For this review, take the finished solid that the model builds, in its own axes (mm). Round coordinates to 2 decimals unless told otherwise and drop trailing zeros. Loops run counter-clockwise (first coordinate to the right, second up) from the corner with the lowest first, then second, coordinate; pieces in that order, holes last.
1. Clearance check with a flat-ended pin moving along its axis: pin 1 Ø4 at (x, y) = (174.625, -53.975) entering from +Z. State where the tip first meets the part, or that it passes through.
2. Draft analysis for pull direction X (two halves, no side actions). For faces 1 (the cylindrical face through (176.971, -13.673, 1.288)), 2 (the flat face through (91, -74, 0)), state which applies: released by +X, released by -X, zero draft, split by the parting line, or undercut.
3. Consider section A-A on y = -95.25. State the section outline as (x, z) points (3 decimals).
4. To check wall thickness, follow line 1 along X through (y, z) = (-53.5, 2.15); line 2 along Y through (x, z) = (11.5, 0.55) (3 decimals); line 3 along Y through (x, z) = (11, 0.95) (3 decimals). State the ranges of each line that lie inside material, in increasing order.
from build123d import *

# Parameters (mm, degrees)
SKETCH1_W                 = 184.15
SKETCH1_H                 = 149.225
BOSS_EXTRUDE1_DEPTH       = 2.54
SKETCH2_R                 = 2.54
CUT_EXTRUDE1_DEPTH        = 2.54
LPATTERN1_COUNT           = 2
LPATTERN1_PITCH           = 50.8
LPATTERN2_COUNT           = 2
LPATTERN2_PITCH           = 41.275
LPATTERN2_COPY_1_SKETCH_R = 2.54
LPATTERN2_COPY_1_DEPTH    = 2.54
SKETCH3_R                 = 2.54
CUT_EXTRUDE2_DEPTH        = 2.54
LPATTERN3_COUNT           = 2
LPATTERN3_PITCH           = 50.8
LPATTERN4_COUNT           = 2
LPATTERN4_PITCH           = 41.275
LPATTERN4_COPY_1_SKETCH_R = 2.54
LPATTERN4_COPY_1_DEPTH    = 2.54
SKETCH5_R                 = 2.54
CUT_EXTRUDE4_DEPTH        = 2.54
LPATTERN7_COUNT           = 2
LPATTERN7_PITCH           = 41.275
LPATTERN8_COUNT           = 2
LPATTERN8_PITCH           = 50.8
LPATTERN8_COPY_1_SKETCH_R = 2.54
LPATTERN8_COPY_1_DEPTH    = 2.54
LPATTERN9_COUNT           = 2
LPATTERN9_PITCH           = 82.55
LPATTERN9_COPY_1_SKETCH_R = 2.54
LPATTERN9_COPY_1_DEPTH    = 2.54
LPATTERN9_COPY_2_SKETCH_R = 2.54
LPATTERN9_COPY_2_DEPTH    = 2.54
LPATTERN9_COPY_3_SKETCH_R = 2.54
LPATTERN9_COPY_3_DEPTH    = 2.54


with BuildPart() as part:
    # Sketch1 → Boss-Extrude1 (new body)
    with BuildSketch(Plane.XY):
        with Locations((92.075, -74.6125)):
            Rectangle(SKETCH1_W, SKETCH1_H)
    extrude(amount=BOSS_EXTRUDE1_DEPTH)

    # Sketch2 → Cut-Extrude1 (cut)
    with BuildSketch(Plane.XY.offset(2.54)):
        with Locations((9.525, -12.7)):
            Circle(SKETCH2_R)
    cut_extrude1 = extrude(amount=-CUT_EXTRUDE1_DEPTH, mode=Mode.SUBTRACT)

    # LPattern1: Cut-Extrude1 ×2
    with Locations(*[(i * LPATTERN1_PITCH, 0, 0) for i in range(1, LPATTERN1_COUNT)]):
        add(cut_extrude1, mode=Mode.SUBTRACT)

    # LPattern2: Cut-Extrude1 ×2
    with Locations(*[(0, -i * LPATTERN2_PITCH, 0) for i in range(1, LPATTERN2_COUNT)]):
        add(cut_extrude1, mode=Mode.SUBTRACT)

    # LPattern2 copy 1 sketch → LPattern2 copy 1 (cut)
    with BuildSketch(Plane(origin=(50.8, -41.275, 2.54), x_dir=(1, 0, 0), z_dir=(0, 0, 1))):
        with Locations((9.525, -12.7)):
            Circle(LPATTERN2_COPY_1_SKETCH_R)
    extrude(amount=-LPATTERN2_COPY_1_DEPTH, mode=Mode.SUBTRACT)

    # Sketch3 → Cut-Extrude2 (cut)
    with BuildSketch(Plane.XY.offset(2.54)):
        with Locations((123.825, -12.7)):
            Circle(SKETCH3_R)
    cut_extrude2 = extrude(amount=-CUT_EXTRUDE2_DEPTH, mode=Mode.SUBTRACT)

    # LPattern3: Cut-Extrude2 ×2
    with Locations(*[(i * LPATTERN3_PITCH, 0, 0) for i in range(1, LPATTERN3_COUNT)]):
        add(cut_extrude2, mode=Mode.SUBTRACT)

    # LPattern4: Cut-Extrude2 ×2
    with Locations(*[(0, -i * LPATTERN4_PITCH, 0) for i in range(1, LPATTERN4_COUNT)]):
        add(cut_extrude2, mode=Mode.SUBTRACT)

    # LPattern4 copy 1 sketch → LPattern4 copy 1 (cut)
    with BuildSketch(Plane(origin=(50.8, -41.275, 2.54), x_dir=(1, 0, 0), z_dir=(0, 0, 1))):
        with Locations((123.825, -12.7)):
            Circle(LPATTERN4_COPY_1_SKETCH_R)
    extrude(amount=-LPATTERN4_COPY_1_DEPTH, mode=Mode.SUBTRACT)

    # Sketch5 → Cut-Extrude4 (cut)
    with BuildSketch(Plane.XY.offset(2.54)):
        with Locations((9.525, -136.525)):
            Circle(SKETCH5_R)
    cut_extrude4 = extrude(amount=-CUT_EXTRUDE4_DEPTH, mode=Mode.SUBTRACT)

    # LPattern7: Cut-Extrude4 ×2
    with Locations(*[(0, i * LPATTERN7_PITCH, 0) for i in range(1, LPATTERN7_COUNT)]):
        add(cut_extrude4, mode=Mode.SUBTRACT)

    # LPattern8: Cut-Extrude4 ×2
    with Locations(*[(i * LPATTERN8_PITCH, 0, 0) for i in range(1, LPATTERN8_COUNT)]):
        add(cut_extrude4, mode=Mode.SUBTRACT)

    # LPattern8 copy 1 sketch → LPattern8 copy 1 (cut)
    with BuildSketch(Plane(origin=(50.8, 41.275, 2.54), x_dir=(1, 0, 0), z_dir=(0, 0, 1))):
        with Locations((9.525, -136.525)):
            Circle(LPATTERN8_COPY_1_SKETCH_R)
    extrude(amount=-LPATTERN8_COPY_1_DEPTH, mode=Mode.SUBTRACT)

    # LPattern9: Cut-Extrude2 ×2
    with Locations(*[(0, -i * LPATTERN9_PITCH, 0) for i in range(1, LPATTERN9_COUNT)]):
        add(cut_extrude2, mode=Mode.SUBTRACT)

    # LPattern9 copy 1 sketch → LPattern9 copy 1 (cut)
    with BuildSketch(Plane(origin=(50.8, -82.55, 2.54), x_dir=(1, 0, 0), z_dir=(0, 0, 1))):
        with Locations((123.825, -12.7)):
            Circle(LPATTERN9_COPY_1_SKETCH_R)
    extrude(amount=-LPATTERN9_COPY_1_DEPTH, mode=Mode.SUBTRACT)

    # LPattern9 copy 2 sketch → LPattern9 copy 2 (cut)
    with BuildSketch(Plane(origin=(0, -123.825, 2.54), x_dir=(1, 0, 0), z_dir=(0, 0, 1))):
        with Locations((123.825, -12.7)):
            Circle(LPATTERN9_COPY_2_SKETCH_R)
    extrude(amount=-LPATTERN9_COPY_2_DEPTH, mode=Mode.SUBTRACT)

    # LPattern9 copy 3 sketch → LPattern9 copy 3 (cut)
    with BuildSketch(Plane(origin=(50.8, -123.825, 2.54), x_dir=(1, 0, 0), z_dir=(0, 0, 1))):
        with Locations((123.825, -12.7)):
            Circle(LPATTERN9_COPY_3_SKETCH_R)
    extrude(amount=-LPATTERN9_COPY_3_DEPTH, mode=Mode.SUBTRACT)


solid = part.part
Resolved:
1. pin 1: passes through
2. face 1: undercut
2. face 2: zero draft
3. outline: (0, 0) - (6.985, 0) - (6.985, 2.54) - (0, 2.54) - close; (12.065, 0) - (57.785, 0) - (57.785, 2.54) - (12.065, 2.54) - close; (62.865, 0) - (121.285, 0) - (121.285, 2.54) - (62.865, 2.54) - close; (126.365, 0) - (172.085, 0) - (172.085, 2.54) - (126.365, 2.54) - close; (177.165, 0) - (184.15, 0) - (184.15, 2.54) - (177.165, 2.54) - close
4. line 1: x = 0 to 7.03, 12.02 to 57.83, 62.82 to 121.33, 126.32 to 172.13, 177.12 to 184.15
4. line 2: y = -149.225 to -138.122, -134.928 to -96.847, -93.653 to -55.572, -52.378 to -14.297, -11.103 to 0
4. line 3: y = -149.225 to -138.593, -134.457 to -97.318, -93.182 to -56.043, -51.907 to -14.768, -10.632 to 0
